Geometry: final body of the model. Coordinates: model frame, mm. Give positions to 0.01 mm unless a question says otherwise; leave off trailing zeros. Write each loop counter-clockwise with the first axis right and the second up, starting at its lowest first coordinate (ties: lowest second). Pieces come first, ordered by that corner, then holes. Notation, with made-up numbers: (88, -34) -> (116, -34) arc R22 ccw to (116, -19) -> close; hole circle Ø5 at (-2.5, -5.75). An arc over 180 degrees is marked (long way). Answer as a JSON object with one key per item and string values.
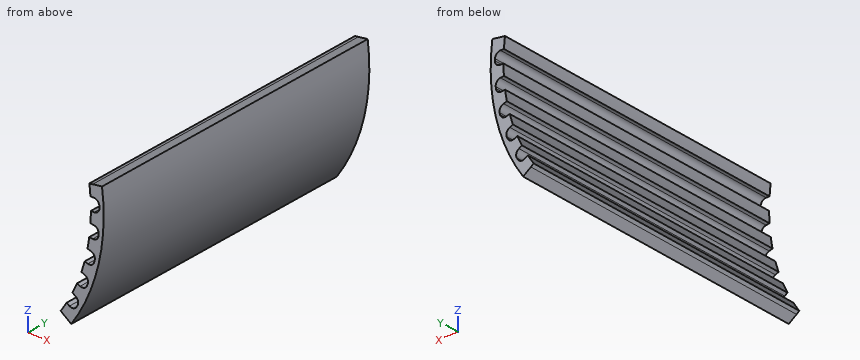
from build123d import *

# Parameters (mm, degrees)
RESSALTO_EXTRUS_O1_DEPTH = 22.5
CORTE_EXTRUS_O1_DEPTH    = 28.741906497


with BuildPart() as part:
    # Esboço1 → Ressalto-extrusão1 (new body)
    with BuildSketch(Plane(origin=(0, 0, 0), x_dir=(1, 0, 0), z_dir=(0, 1, 0))):
        with BuildLine():
            Line((10.760467264, 7.350777988), (10.969182874, 7.504560719))
            ThreePointArc((10.969182874, 7.504560719), (11.122613734, 7.740848698), (11.082224189, 8.019670724))
            Line((11.082224189, 8.019670724), (11.341808671, 8.207519484))
            ThreePointArc((11.341808671, 8.207519484), (13.61934662, 3.242436992), (13.823462506, -2.216277139))
            Line((13.823462506, -2.216277139), (13.507778422, -2.165664391))
            ThreePointArc((13.507778422, -2.165664391), (13.420279696, -1.89483606), (13.174835153, -1.750749321))
            Line((13.174835153, -1.750749321), (12.919194973, -1.707628189))
            ThreePointArc((12.919194973, -1.707628189), (12.966114499, -1.304403152), (13.000451936, -0.899912346))
            Line((13.000451936, -0.899912346), (13.259558649, -0.908575229))
            ThreePointArc((13.259558649, -0.908575229), (13.545442602, -0.801602223), (13.67263107, -0.524120778))
            ThreePointArc((13.67263107, -0.524120778), (13.675032192, -0.457206207), (13.677105833, -0.390280687))
            ThreePointArc((13.677105833, -0.390280687), (13.568735109, -0.104923638), (13.290634577, 0.020905426))
            Line((13.290634577, 0.020905426), (13.031527865, 0.029568308))
            ThreePointArc((13.031527865, 0.029568308), (13.024284113, 0.435449325), (13.004401826, 0.840907789))
            Line((13.004401826, 0.840907789), (13.262351305, 0.866857746))
            ThreePointArc((13.262351305, 0.866857746), (13.53142635, 1.010980886), (13.62049532, 1.302939063))
            ThreePointArc((13.62049532, 1.302939063), (13.613956179, 1.369576627), (13.607091018, 1.436181392))
            ThreePointArc((13.607091018, 1.436181392), (13.461652861, 1.704547935), (13.169262312, 1.792187114))
            Line((13.169262312, 1.792187114), (12.911312833, 1.766237157))
            ThreePointArc((12.911312833, 1.766237157), (12.850035069, 2.167531198), (12.776287858, 2.566721906))
            Line((12.776287858, 2.566721906), (13.028476989, 2.626821624))
            ThreePointArc((13.028476989, 2.626821624), (13.275941474, 2.805523017), (13.325301509, 3.106747926))
            ThreePointArc((13.325301509, 3.106747926), (13.309938795, 3.171919333), (13.294257343, 3.23701478))
            ThreePointArc((13.294257343, 3.23701478), (13.114347099, 3.48360181), (12.812884249, 3.531487182))
            Line((12.812884249, 3.531487182), (12.560695118, 3.471387463))
            ThreePointArc((12.560695118, 3.471387463), (12.446476845, 3.860933427), (12.32018073, 4.246732809))
            Line((12.32018073, 4.246732809), (12.562109192, 4.339909808))
            ThreePointArc((12.562109192, 4.339909808), (12.783547108, 4.550000523), (12.792317376, 4.855116798))
            ThreePointArc((12.792317376, 4.855116798), (12.768405238, 4.917659063), (12.744187329, 4.980083563))
            ThreePointArc((12.744187329, 4.980083563), (12.533015503, 5.200490728), (12.227859963, 5.207767777))
            Line((12.227859963, 5.207767777), (11.985931502, 5.114590777))
            ThreePointArc((11.985931502, 5.114590777), (11.820810947, 5.485437206), (11.644219685, 5.850960664))
            Line((11.644219685, 5.850960664), (11.871570259, 5.975552199))
            ThreePointArc((11.871570259, 5.975552199), (12.06303004, 6.213283162), (12.031054037, 6.516845996))
            ThreePointArc((12.031054037, 6.516845996), (11.999019187, 6.575643051), (11.966696991, 6.634282636))
            ThreePointArc((11.966696991, 6.634282636), (11.728031948, 6.824576766), (11.424629227, 6.791115632))
            Line((11.424629227, 6.791115632), (11.197278653, 6.666524097))
            ThreePointArc((11.197278653, 6.666524097), (10.984202397, 7.012053229), (10.760467264, 7.350777988))
        make_face()
    extrude(amount=RESSALTO_EXTRUS_O1_DEPTH)

    # Esboço2 → Corte-extrusão1 (cut, through all)
    with BuildSketch(Plane(origin=(0, 22.5, 0), x_dir=(1, 0, 0), z_dir=(0, 1, 0))):
        with BuildLine():
            Line((13.174835153, -1.750749321), (13.874709853, -1.868803493))
            ThreePointArc((13.874709853, -1.868803493), (13.850175901, -2.042701034), (13.823462506, -2.216277139))
            Line((13.823462506, -2.216277139), (13.507778422, -2.165664391))
            ThreePointArc((13.507778422, -2.165664391), (13.420279696, -1.89483606), (13.174835153, -1.750749321))
        make_face()
        with BuildLine():
            Line((10.969182874, 7.504560719), (11.554630395, 7.905094334))
            ThreePointArc((11.554630395, 7.905094334), (11.449218127, 8.057009637), (11.341808671, 8.207519484))
            Line((11.341808671, 8.207519484), (11.082224189, 8.019670724))
            ThreePointArc((11.082224189, 8.019670724), (11.122613734, 7.740848698), (10.969182874, 7.504560719))
        make_face()
    extrude(amount=-CORTE_EXTRUS_O1_DEPTH, mode=Mode.SUBTRACT)


solid = part.part
Q1. Cut plane A-A (z = -3.75). Return the cut outline in (x, y), and give its area (3 significant figures).
Values:
{"outline": "(12.48, 0) -> (13.49, 0) -> (13.49, 22.5) -> (12.48, 22.5) -> close", "area": "22.7 mm²"}
Q2. First-contact query: P1, Ø5, axis at y = 5.5, z = -2, coming from the -X side; P2, Ø1.5, axis at x = 13, z = 0, coming from the +Y side; P3, Ø1, axis at x = 12.5, y = 15.5, coming from the +Z side. Flat tips, straight axial feed; report the tip coordinate or a pass-through.
Values:
{"P1": "x = 12.32", "P2": "y = 22.5", "P3": "z = 1.72"}
Q3. Material intervals for L1, parallel to X at y = 1.5, z = -6.75; L2, parallel to Z at x = 11.5, y = 15; L3, parallel to X at y = 2, z = -1, sorted ascending. Write a range as from..to.
Values:
{"L1": "11.15..11.35, 11.87..12.27", "L2": "-7.87..-6.82", "L3": "13.52..13.96"}
